```python
from build123d import *

# Parameters (mm, degrees)
SKETCH1_W           = 76
SKETCH1_H           = 76
BOSS_EXTRUDE1_DEPTH = 4.5
SKETCH2_R           = 3.1
SKETCH2_R_2         = 2.5
SKETCH2_R_3         = 7
SKETCH2_R_4         = 1.575
CUT_EXTRUDE1_DEPTH  = 108.574392864
FILLET1_R           = 10
SKETCH3_R           = 7.25
CUT_EXTRUDE2_DEPTH  = 3.8
SKETCH4_R           = 4
CUT_EXTRUDE3_DEPTH  = 2
FILLET2_R           = 3
BOSS_EXTRUDE2_START = 2.5
SKETCH6_R           = 30
SKETCH6_R_2         = 2.5
SKETCH6_R_3         = 3.1
SKETCH6_R_4         = 4
BOSS_EXTRUDE2_DEPTH = 2.5


with BuildPart() as part:
    # Sketch1 → Boss-Extrude1 (new body)
    with BuildSketch(Plane.XY):
        with Locations((38, 38)):
            Rectangle(SKETCH1_W, SKETCH1_H)
    extrude(amount=BOSS_EXTRUDE1_DEPTH)

    # Sketch2 → Cut-Extrude1 (cut, through all)
    with BuildSketch(Plane.XY.offset(4.5)):
        with Locations((55.67766953, 55.67766953)):
            Circle(SKETCH2_R)
        with Locations((20.32233047, 55.67766953)):
            Circle(SKETCH2_R)
        with Locations((20.32233047, 20.32233047)):
            Circle(SKETCH2_R)
        with Locations((55.67766953, 20.32233047)):
            Circle(SKETCH2_R)
        with Locations((38, 38)):
            Circle(SKETCH2_R_2)
        with Locations((66.213560569, 66.354981926)):
            Circle(SKETCH2_R_3)
        with Locations((42.808326112, 58.647518011)):
            Circle(SKETCH2_R_4)
        with Locations((58.506096654, 42.949747468)):
            Circle(SKETCH2_R_4)
        with Locations((17.352481989, 33.191673888)):
            Circle(SKETCH2_R_4)
        with Locations((9.645018074, 9.786439431)):
            Circle(SKETCH2_R_3)
        with Locations((33.050252532, 17.493903346)):
            Circle(SKETCH2_R_4)
    extrude(amount=-CUT_EXTRUDE1_DEPTH, mode=Mode.SUBTRACT)

    # Fillet1
    fillet1_edges = [part.edges().sort_by_distance(p)[0] for p in [
        (0, 76, 2.25),
        (76, 76, 2.25),
        (76, 0, 2.25),
        (0, 0, 2.25),
    ]]
    fillet(fillet1_edges, radius=FILLET1_R)

    # Sketch3 → Cut-Extrude2 (cut)
    with BuildSketch(Plane(origin=(0, 0, 0), x_dir=(-1, 0, 0), z_dir=(0, 0, -1))):
        with Locations((-55.67766953, 55.67766953)):
            Circle(SKETCH3_R)
        with Locations((-20.32233047, 55.67766953)):
            Circle(SKETCH3_R)
        with Locations((-55.67766953, 20.32233047)):
            Circle(SKETCH3_R)
        with Locations((-20.32233047, 20.32233047)):
            Circle(SKETCH3_R)
    extrude(amount=-CUT_EXTRUDE2_DEPTH, mode=Mode.SUBTRACT)

    # Sketch4 → Cut-Extrude3 (cut)
    with BuildSketch(Plane.XY.offset(4.5)):
        with Locations((58.506096654, 42.949747468)):
            Circle(SKETCH4_R)
        with Locations((33.050252532, 17.493903346)):
            Circle(SKETCH4_R)
        with Locations((17.352481989, 33.191673888)):
            Circle(SKETCH4_R)
        with Locations((42.808326112, 58.647518011)):
            Circle(SKETCH4_R)
    extrude(amount=-CUT_EXTRUDE3_DEPTH, mode=Mode.SUBTRACT)

    # Fillet2
    # the kernel refuses this fillet: 3 mm, written as the material it takes off along each edge
    with BuildSketch(Plane(origin=(66.213560569, 66.354981926, 0), x_dir=(1, 0, 0), z_dir=(0, -1, 0))) as fillet2_piece_1:
        with BuildLine():
            CenterArc((7 + FILLET2_R, FILLET2_R), FILLET2_R, 180, 90)
            Line((7, FILLET2_R), (7, 0))
            Line((7, 0), (7 + FILLET2_R, 0))
        make_face()
    revolve(axis=Axis((66.213560569, 66.354981926, 0), (0, 0, 1)), mode=Mode.SUBTRACT)
    with BuildSketch(Plane(origin=(9.645018074, 9.786439431, 0), x_dir=(1, 0, 0), z_dir=(0, -1, 0))) as fillet2_piece_2:
        with BuildLine():
            CenterArc((7 + FILLET2_R, FILLET2_R), FILLET2_R, 180, 90)
            Line((7, FILLET2_R), (7, 0))
            Line((7, 0), (7 + FILLET2_R, 0))
        make_face()
    revolve(axis=Axis((9.645018074, 9.786439431, 0), (0, 0, 1)), mode=Mode.SUBTRACT)

    # Sketch6 → Boss-Extrude2 (add)
    with BuildSketch(Plane.XY.offset(4.5).offset(BOSS_EXTRUDE2_START)):
        with Locations((38, 38)):
            Circle(SKETCH6_R)
        with Locations((38, 38)):
            Circle(SKETCH6_R_2, mode=Mode.SUBTRACT)
        with Locations((55.67766953, 55.67766953)):
            Circle(SKETCH6_R_3, mode=Mode.SUBTRACT)
        with Locations((55.67766953, 20.32233047)):
            Circle(SKETCH6_R_3, mode=Mode.SUBTRACT)
        with Locations((20.32233047, 55.67766953)):
            Circle(SKETCH6_R_3, mode=Mode.SUBTRACT)
        with Locations((58.506096654, 42.949747468)):
            Circle(SKETCH6_R_4, mode=Mode.SUBTRACT)
        with Locations((42.808326112, 58.647518011)):
            Circle(SKETCH6_R_4, mode=Mode.SUBTRACT)
        with Locations((33.050252532, 17.493903346)):
            Circle(SKETCH6_R_4, mode=Mode.SUBTRACT)
        with Locations((17.352481989, 33.191673888)):
            Circle(SKETCH6_R_4, mode=Mode.SUBTRACT)
        with Locations((20.32233047, 20.32233047)):
            Circle(SKETCH6_R_3, mode=Mode.SUBTRACT)
    extrude(amount=-BOSS_EXTRUDE2_DEPTH)


solid = part.part
```
Model file for the job. Use its own axes, mm. A direction names the side the tool comes from. Coordinates: 2 decimals unless noted, no trailing zeros. Loops run counter-clockwise (first coordinate to the right, second up) from the corner with the lowest first, then second, coordinate; pieces in that order, holes last. Notation, with made-up numbers: M 15.25,50 L 35.25,50 A13 ccw 35.25,74 Z; hole C -25.5,44.25 d11. An arc over 180 degrees is marked long. Use CSV: the item, a comma, the result in double quotes. Start each with the question number.
1. Flat gauge pins, fed straight in: pin 1 (3.5 mm diameter, centred on x = 20.32, y = 55.68, fed in from +Z); pin 2 (8.5 mm diameter, centred on x = 55.68, y = 55.68, fed in from -Z); pin 3 (16 mm diameter, centred on x = 66.21, y = 66.35, fed in from +Z); pin 4 (2.5 mm diameter, centred on x = 57, y = 43, fed in from +Z). Where does each tip first touch, or does it go through?
2. Band-saw the part on C-C, the plane x = 43. List the corners of the cut face in (y, z).
3. Band-saw the part on A-A, the plane x = 22.5. List the corners of the cut face in (y, z), then the cut area to 3 significant figures.
4. Tool access for faces 1 (the cylindrical face through (31.477, 17.563, 1.268)), 2 (the cylindrical face through (25.67, 25.22, 1.87)), 3 (the flat face through (21, 64, 4.5)): list every direction of +Z, -Z, +X, -X, +Y, -Y with a clear straight run to the whole face (end or side of a thin tool).
5. Probe probe 1 along X at (y, z) = (55, 5); probe 2 along X at (y, z) = (40, 5.75); probe 3 along X at (y, z) = (25, 2.5). List the from-to ranges inside material, lowest first. Write a range as [from, to].
6. Band-saw the part on B-B, the plane z = 5.5. Give the number of separate pieces and of enclosed holes in the cut face, then the cut area to 3 significant figures.
Entries:
1,pin 1,"passes through"
1,pin 2,"stops at z = 3.8"
1,pin 3,"stops at z = 4.5"
1,pin 4,"stops at z = 2.5"
2,outline,"M 0,0 L 57.08,0 L 57.08,2.5 L 54.65,2.5 L 54.65,7 L 8.42,7 L 8.42,4.5 L 0,4.5 Z; M 60.21,0 L 76,0 L 76,4.5 L 67.58,4.5 L 67.58,7 L 62.64,7 L 62.64,2.5 L 60.21,2.5 Z"
3,outline,"M 0,0 L 13.41,0 L 13.41,3.8 L 18.12,3.8 L 18.12,7 L 12.31,7 L 12.31,4.5 L 0,4.5 Z; M 22.53,3.8 L 27.24,3.8 L 27.24,0 L 48.76,0 L 48.76,3.8 L 53.47,3.8 L 53.47,7 L 22.53,7 Z; M 57.88,3.8 L 62.59,3.8 L 62.59,0 L 76,0 L 76,4.5 L 63.69,4.5 L 63.69,7 L 57.88,7 Z"
3,area,"337 mm2"
4,face 1,"+Z, -Z"
4,face 2,"-Z"
4,face 3,"+Z"
5,probe 1,"x = [13.28, 17.3], [23.35, 41.17], [44.45, 52.65], [58.7, 62.72]"
5,probe 2,"x = [8.07, 36.5], [39.5, 55.8], [61.21, 67.93]"
5,probe 3,"x = [0, 14.78], [25.86, 50.14], [61.22, 76]"
6,separate pieces,"1"
6,enclosed holes,"9"
6,area,"2,490 mm2"
